For this review, take the finished solid that the model builds, in its own axes (mm). Face numbers are marked on the shaded views. A direction names the side the tool comes from. Give positions to 0.01 mm unless a question says otherwise; leave off trailing zeros. Order: outer loops, then holes, each group sorted by start corner. A loop starts at its lowest first (then second) coordinate and runs counter-clockwise, first axis right, second up.
Item 1: Consider section A-A (z = 223). Give the boundary of the cut face in (x, y) (3 decimals), plus the area to 3 significant figures.
Item 2: For P1, Ø9, axis at y = -1.5, z = -15, coming from the +X side; P2, Ø18, axis at x = -9.9, y = -1.49, coming from the -Z side; P3, Ø10, axis at x = -19.5, z = 196.5, coming from the -Y side (3 decimals); P4, Ø10.5, axis at y = 0.5, z = 197, coming from the +X side, all flat-tipped, find the tip position at first contact; note any pin that passes through.
Item 3: For probe 1 along Y at (x, z) = (-7, -12.7); probe 2 along Z at (x, y) = (-0.5, -3); probe 3 along Z at (x, y) = (7.5, -53), list the stretches that pass through material, from the lowest coordinate up.
Item 4: Machinability: for the marked faces 1, 2, 3, 4 and 5, which of the approach directions +Z, -Z, +X, -X, +Y, -Y give a long, thin tool a straight path to every point of the face, cutting with its end or side? Answer none if there is none.
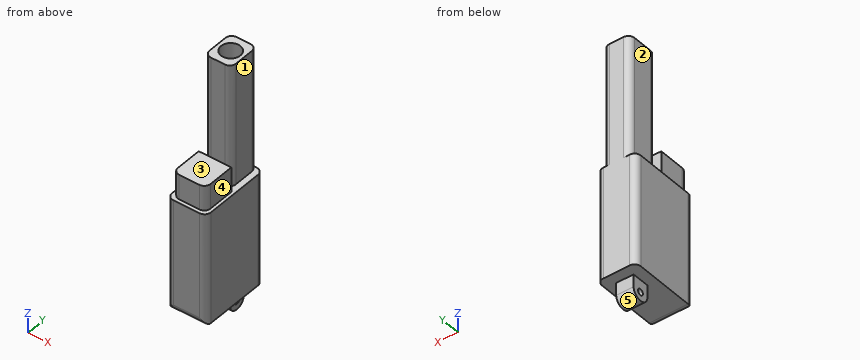
Autodesk Inventor part; units mm, degrees
ref_plane "YZ Plane" through (0, 0, 0) normal (1, 0, 0) x (0, 1, 0)
ref_plane "XZ Plane" through (0, 0, 0) normal (0, 1, 0) x (-1, 0, 0)
ref_plane "XY Plane" through (0, 0, 0) normal (0, 0, 1) x (1, 0, 0)
sketch "Sketch1" plane through (0, 0, 0) normal (0, 0, 1) x (1, 0, 0)
  line L0 (-29.7166, 15.149) -> (9.9074, 15.149)
  line L1 (9.9074, 15.149) -> (9.9074, -58.765)
  line L2 (9.9074, -58.765) -> (-29.7166, -58.765)
  line L3 (-29.7166, -58.765) -> (-29.7166, 15.149)
  point P0 (0, 0)
  dimension "d0" = 39.624
  dimension "d1" = 73.914
extrude "Extrusion1" add sketch "Sketch1" along normal blind 76.2
sketch "Sketch2" plane through (0, 0, 76.2) normal (0, 0, 1) x (1, 0, 0)
  line L0 (9.9074, 15.149) -> (9.9074, -58.765)
  line L1 (-29.7166, 15.149) -> (9.9074, 15.149)
  line L2 (9.9074, 15.149) -> (9.9074, -24.475)
  line L3 (9.9074, -24.475) -> (-29.7166, -24.475)
  line L4 (-29.7166, -24.475) -> (-29.7166, 15.149)
  line L5 (-29.7166, -24.475) -> (-23.3666, -24.475)
  line L6 (-23.3666, -24.475) -> (-23.3666, -18.125)
  line L7 (-23.3666, -18.125) -> (-29.7166, -18.125)
  line L8 (-29.7166, -18.125) -> (-29.7166, -24.475)
  line L9 (-23.3666, -18.125) -> (3.5574, -18.125)
  line L10 (3.5574, -18.125) -> (3.5574, 15.149)
  line L11 (3.5574, 15.149) -> (-23.3666, 15.149)
  line L12 (-23.3666, 15.149) -> (-23.3666, -18.125)
  point P0 (0, 0)
  dimension "d4" = 39.624
  dimension "d5" = 6.35
  dimension "d6" = 6.35
  dimension "d7" = 26.924
extrude "Extrusion2" add sketch "Sketch2" along normal blind 162.56 contours L10 L9 L12 L1
sketch "Sketch3" plane through (0, 0, 238.76) normal (0, 0, 1) x (1, 0, 0)
  line L0 (-23.3666, 15.149) -> (3.5574, -18.125)
  line L1 (3.5574, 15.149) -> (-23.3666, -18.125)
  circle A0 centre (-9.9046, -1.488) radius 9.906
  point P0 (0, 0)
  dimension "d10" = 19.812
extrude "Extrusion3" cut sketch "Sketch3" against normal blind 203.2
sketch "Sketch4" plane through (0, 0, 76.2) normal (0, 0, 1) x (1, 0, 0)
  line L0 (3.5574, 15.149) -> (3.5574, -18.125)
  line L1 (3.5574, -18.125) -> (-23.3666, -18.125)
  line L2 (-23.3666, -18.125) -> (-23.3666, 15.149)
  line L3 (-29.7166, 15.149) -> (-23.3666, 15.149)
  line L4 (-29.7166, -58.765) -> (-29.7166, 15.149)
  line L5 (9.9074, -58.765) -> (-29.7166, -58.765)
  line L6 (9.9074, 15.149) -> (9.9074, -58.765)
  line L7 (3.5574, 15.149) -> (9.9074, 15.149)
  point P0 (0, 0)
extrude "Extrusion4" cut sketch "Sketch4" against normal blind 25.4
sketch "Sketch5" plane through (0, 0, 50.8) normal (0, 0, 1) x (1, 0, 0)
  line L0 (-26.5416, -21.808) -> (6.7324, -21.808)
  line L1 (6.7324, -21.808) -> (6.7324, -55.082)
  line L2 (6.7324, -55.082) -> (-26.5416, -55.082)
  line L3 (-26.5416, -55.082) -> (-26.5416, -21.808)
  point P0 (0, 0)
  dimension "d15" = 33.274
extrude "Extrusion5" add sketch "Sketch5" along normal blind 88.9
sketch "Sketch6" plane through (0, 0, 50.8) normal (0, 0, 1) x (1, 0, 0)
  line L0 (6.7324, -21.808) -> (6.7324, -55.082)
  line L1 (6.7324, -55.082) -> (-26.5416, -55.082)
  line L2 (-26.5416, -55.082) -> (-26.5416, -21.808)
  line L3 (-26.5416, -21.808) -> (6.7324, -21.808)
  line L4 (3.5574, -18.125) -> (-23.3666, -18.125)
  line L5 (-23.3666, -18.125) -> (-23.3666, 15.149)
  line L6 (-29.7166, 15.149) -> (-23.3666, 15.149)
  line L7 (-29.7166, -58.765) -> (-29.7166, 15.149)
  line L8 (9.9074, -58.765) -> (-29.7166, -58.765)
  line L9 (9.9074, 15.149) -> (9.9074, -58.765)
  line L10 (3.5574, 15.149) -> (9.9074, 15.149)
  line L11 (3.5574, 15.149) -> (3.5574, -18.125)
  point P0 (0, 0)
extrude "Extrusion6" add sketch "Sketch6" along normal blind 25.4
sketch "Sketch7" plane through (0, 0, 0) normal (0, 0, -1) x (-1, 0, 0)
  line L0 (-9.9074, 15.149) -> (-9.9074, -58.765)
  line L1 (29.7166, -58.765) -> (29.7166, 15.149)
  line L2 (-9.9074, 15.149) -> (29.7166, -24.475)
  line L3 (-9.9074, 15.149) -> (46.1294, 15.149) construction
  line L4 (29.7166, 15.149) -> (-9.9074, -24.475)
  line L5 (1.0146, 4.227) -> (18.7946, 4.227)
  line L6 (1.0146, 4.227) -> (18.7946, 4.227)
  line L7 (18.7946, 4.227) -> (18.7946, -13.553)
  line L8 (18.7946, -13.553) -> (1.0146, -13.553)
  line L9 (1.0146, -13.553) -> (1.0146, 4.227)
  point P0 (0, 0)
  dimension "d20" = 45
  dimension "d21" = 17.78
extrude "Extrusion7" add sketch "Sketch7" along normal blind 12.7 contours L5 L4 L2 | L2 L4 L9 | L4 L2 L8 | L4 L7 L2
sketch "Sketch8" plane through (-18.7946, -13.553, 0) normal (-1, 0, 0) x (0, 0, 1)
  line L0 (-12.7, 17.78) -> (-12.7, 0)
  circle A0 centre (-12.7, 8.89) radius 3.175
  point P0 (0, 13.553)
  dimension "d24" = 6.35
extrude "Extrusion8" cut sketch "Sketch8" against normal blind 25.4
sketch "Sketch9" plane through (-1.0146, -13.553, 0) normal (1, 0, 0) x (0, 0, -1)
  arc A0 (12.7, 12.065) -> (12.7, 5.715) centre (12.7, 8.89) ccw
  circle A1 centre (12.7, 8.89) radius 3.175
  circle A2 centre (12.7, 8.89) radius 8.89
  point P0 (0, 13.553)
extrude "Extrusion9" add sketch "Sketch9" against normal blind 17.78
sketch "Sketch10" plane through (0, 0, 76.2) normal (0, 0, 1) x (1, 0, 0)
  line L0 (-26.5416, -55.082) -> (6.7324, -55.082)
  line L1 (-26.5416, -21.808) -> (-26.5416, -55.082)
  line L2 (6.7324, -21.808) -> (-26.5416, -21.808)
  line L3 (6.7324, -55.082) -> (6.7324, -21.808)
  line L4 (3.5574, -18.125) -> (3.5574, 15.149)
  line L5 (-23.3666, -18.125) -> (3.5574, -18.125)
  line L6 (-23.3666, 15.149) -> (-23.3666, -18.125)
  line L7 (-29.7166, 15.149) -> (-23.3666, 15.149)
  line L8 (-29.7166, -58.765) -> (-29.7166, 15.149)
  line L9 (9.9074, -58.765) -> (-29.7166, -58.765)
  line L10 (9.9074, 15.149) -> (9.9074, -58.765)
  line L11 (3.5574, 15.149) -> (9.9074, 15.149)
  point P0 (0, 0)
extrude "Extrusion10" add sketch "Sketch10" along normal blind 38.1
fillet "Fillet1" radius 6.35 11 edges at (9.9074, 15.149, 57.15) (-29.7166, 15.149, 57.15) (9.9074, -58.765, 57.15) (-29.7166, -58.765, 57.15) (-26.5416, -55.082, 127) (6.7324, -55.082, 127) (-9.9046, -58.765, 0) (-23.3666, 15.149, 176.53) (3.5574, 15.149, 176.53) (-23.3666, -18.125, 176.53) (3.5574, -18.125, 176.53)
properties part number "linac body"
Resolved:
1. outline: (-23.367, -11.775) arc R6.35 ccw to (-17.017, -18.125) - (-2.793, -18.125) arc R6.35 ccw to (3.557, -11.775) - (3.557, 8.799) arc R6.35 ccw to (-2.793, 15.149) - (-17.017, 15.149) arc R6.35 ccw to (-23.367, 8.799) - close; hole circle Ø19.812 at (-9.905, -1.488)
1. area: 553 mm2
2. P1: stops at x = -1.01
2. P2: stops at z = -21.59
2. P3: stops at y = -18.125
2. P4: stops at x = 3.56
3. probe 1: y = -13.55 to -7.84, -1.49 to 4.23
3. probe 2: z = 0 to 35.56
3. probe 3: z = 0.03 to 114.3
4. face 1: +Z, +X, +Y
4. face 2: +Z, -X, +Y
4. face 3: +Z, +X, -X, -Y
4. face 4: +Z, +X, +Y, -Y
4. face 5: -Z, +X, -X
